Design review of the part built by this model. Coordinates are the model's own, in mm. A direction names the side the tool comes from. Coordinates: 2 decimals unless noted, no trailing zeros. Write each loop counter-clockwise with the first axis right and the second up, starting at its lowest first coordinate (ties: lowest second). Pieces come first, ordered by that corner, then holes. Notation, with made-up numbers: (24.5, 31) - (68.5, 31) arc R26 ccw to (68.5, 55) - close; hole circle Ø6 at (20, -32.75). An arc over 180 degrees is marked (long way). One line per item, written item: value.
from build123d import *

# Parameters (mm, degrees)
BOSS_EXTRUDE1_DEPTH                           = 3.175
SKETCH2_R                                     = 7.9375
CUT_EXTRUDE1_DEPTH                            = 3.175
CSK_FOR_4_FLAT_HEAD_SOCKET_CAP_SCREW1_A_COUNT = 2
CSK_FOR_4_FLAT_HEAD_SOCKET_CAP_SCREW1_A_PITCH = 44.901280605
CSK_FOR_4_FLAT_HEAD_SOCKET_CAP_SCRE_2_COUNT   = 2
CSK_FOR_4_FLAT_HEAD_SOCKET_CAP_SCRE_2_PITCH   = 44.901280605
CSK_FOR_4_FLAT_HEAD_SOCKET_CAP_SCRE_3_COUNT   = 2
CSK_FOR_4_FLAT_HEAD_SOCKET_CAP_SCRE_3_PITCH   = 81.964210025
CSK_FOR_4_FLAT_HEAD_SOCKET_CAP_SCRE_4_COUNT   = 2
CSK_FOR_4_FLAT_HEAD_SOCKET_CAP_SCRE_4_PITCH   = 81.964210025
SKETCH6_R                                     = 11.1125
SKETCH6_R_2                                   = 7.9375
BOSS_EXTRUDE2_DEPTH                           = 6.096
SKETCH7_R                                     = 8.73125
SKETCH7_R_2                                   = 6.35
BOSS_EXTRUDE3_DEPTH                           = 3.556
CUT_EXTRUDE2_START                            = -2.032
SKETCH8_R                                     = 6.35
CUT_EXTRUDE2_DEPTH                            = 2.032
FILLET1_R                                     = 3.175


with BuildPart() as part:
    # Sketch1 → Boss-Extrude1 (new body)
    with BuildSketch(Plane.XY):
        with BuildLine():
            Line((-34.925, 5.715), (-34.925, -41.275))
            Line((-34.925, -41.275), (34.925, -41.275))
            Line((34.925, -41.275), (34.925, 5.715))
            ThreePointArc((34.925, 5.715), (0, 40.64), (-34.925, 5.715))
        make_face()
    extrude(amount=BOSS_EXTRUDE1_DEPTH)

    # Sketch2 → Cut-Extrude1 (cut)
    with BuildSketch(Plane.XY.offset(3.175)):
        with Locations((0, 5.715)):
            Circle(SKETCH2_R)
    extrude(amount=-CUT_EXTRUDE1_DEPTH, mode=Mode.SUBTRACT)

    # Sketch5 → CSK for #4 Flat Head Socket Cap Screw1 (revolve, cut)
    with BuildSketch(Plane(origin=(0, 37.465, 3.175), x_dir=(0, -1, 0), z_dir=(1, 0, 0))):
        Polygon((0, 0), (0, 3.175), (1.63195, 3.175), (1.63195, 1.848124365), (3.2385, 0), align=None)
    csk_for_4_flat_head_socket_cap_screw1 = revolve(axis=Axis((0, 37.465, 9.525), (0, 0, -1)), mode=Mode.SUBTRACT)

    # CSK for #4 Flat Head Socket Cap Screw1 a: CSK for #4 Flat Head Socket Cap Screw1 ×2
    with Locations(*[Vector(-0.7071067811865475, -0.7071067811865476, 0) * (i * CSK_FOR_4_FLAT_HEAD_SOCKET_CAP_SCREW1_A_PITCH) for i in range(1, CSK_FOR_4_FLAT_HEAD_SOCKET_CAP_SCREW1_A_COUNT)]):
        add(csk_for_4_flat_head_socket_cap_screw1, mode=Mode.SUBTRACT)

    # CSK for _4 Flat Head Socket Cap Scre 2: CSK for #4 Flat Head Socket Cap Screw1 ×2
    with Locations(*[Vector(0.7071067811865475, -0.7071067811865477, 0) * (i * CSK_FOR_4_FLAT_HEAD_SOCKET_CAP_SCRE_2_PITCH) for i in range(1, CSK_FOR_4_FLAT_HEAD_SOCKET_CAP_SCRE_2_COUNT)]):
        add(csk_for_4_flat_head_socket_cap_screw1, mode=Mode.SUBTRACT)

    # CSK for _4 Flat Head Socket Cap Scre 3: CSK for #4 Flat Head Socket Cap Screw1 ×2
    with Locations(*[Vector(0.3873641921317683, -0.9219267772736089, 0) * (i * CSK_FOR_4_FLAT_HEAD_SOCKET_CAP_SCRE_3_PITCH) for i in range(1, CSK_FOR_4_FLAT_HEAD_SOCKET_CAP_SCRE_3_COUNT)]):
        add(csk_for_4_flat_head_socket_cap_screw1, mode=Mode.SUBTRACT)

    # CSK for _4 Flat Head Socket Cap Scre 4: CSK for #4 Flat Head Socket Cap Screw1 ×2
    with Locations(*[Vector(-0.3873641921317683, -0.9219267772736089, 0) * (i * CSK_FOR_4_FLAT_HEAD_SOCKET_CAP_SCRE_4_PITCH) for i in range(1, CSK_FOR_4_FLAT_HEAD_SOCKET_CAP_SCRE_4_COUNT)]):
        add(csk_for_4_flat_head_socket_cap_screw1, mode=Mode.SUBTRACT)

    # Sketch6 → Boss-Extrude2 (add)
    with BuildSketch(Plane(origin=(0, 0, 0), x_dir=(-1, 0, 0), z_dir=(0, 0, -1))):
        with Locations(Location((0, 5.715, 0), (0, 0, 180))):
            Circle(SKETCH6_R)
        with Locations(Location((0, 5.715, 0), (0, 0, 180))):
            Circle(SKETCH6_R_2, mode=Mode.SUBTRACT)
    extrude(amount=BOSS_EXTRUDE2_DEPTH)

    # Sketch7 → Boss-Extrude3 (add)
    with BuildSketch(Plane(origin=(0, 0, 0), x_dir=(-1, 0, 0), z_dir=(0, 0, -1))):
        with Locations(Location((15.875, -25.393519733, 0), (0, 0, 180))):
            Circle(SKETCH7_R)
        with Locations((15.875, -25.393519733)):
            Circle(SKETCH7_R_2, mode=Mode.SUBTRACT)
    extrude(amount=BOSS_EXTRUDE3_DEPTH)

    # Sketch8 → Cut-Extrude2 (cut)
    with BuildSketch(Plane(origin=(0, 0, 0), x_dir=(-1, 0, 0), z_dir=(0, 0, -1)).offset(CUT_EXTRUDE2_START)):
        with Locations((15.875, -25.393519733)):
            Circle(SKETCH8_R)
    extrude(amount=CUT_EXTRUDE2_DEPTH, mode=Mode.SUBTRACT)

    # Fillet1
    fillet1_edges = [part.edges().sort_by_distance(p)[0] for p in [
        (-11.1125, 5.715, 0),
        (-24.60625, -25.393519733, 0),
    ]]
    fillet(fillet1_edges, radius=FILLET1_R)


solid = part.part
1. Wall thickness on line 1 along X through (y, z) = (-38.1, 0.7) (3 decimals); line 2 along Y through (x, z) = (0, 0.5) (1 decimal); line 3 along Y through (x, z) = (1, 1.75) (3 decimals): over which ranges is each line inside the solid? List them lowest first.
Answer block:
line 1: x = -34.925 to -33.382, -30.118 to 30.118, 33.382 to 34.925
line 2: y = -41.3 to -2.2, 13.7 to 35.8, 39.1 to 40.6
line 3: y = -41.275 to -2.159, 13.589 to 35.733, 39.197 to 40.626
2. Consider section B-B, the plane y = -12. Write out the cut boundary in (x, z) (3 decimals).
Answer block:
outline: (-34.925, 0) - (34.925, 0) - (34.925, 3.175) - (-34.925, 3.175) - close
3. Consider section C-C, the plane y = 24. Write out the cut boundary in (x, z) (3 decimals).
Answer block:
outline: (-29.756, 0) - (29.756, 0) - (29.756, 3.175) - (-29.756, 3.175) - close
4. Mouldability with a two-part tool opening along Y and no side actions: class faces 4 (the face through (-33.468, 5.941, 1.442)), 5 (the face through (0, -41.275, 2)), 6 (the face through (0, -9, 3.175)) as released by +Y, released by -Y, zero draft, split by the parting line, or undercut.
Answer block:
face 4: undercut
face 5: released by -Y
face 6: zero draft
5. Insertion check: pin 1 Ø6.5 at (x, y) = (-13.5, -27) entering from -Z; pin 2 Ø1.5 at (x, y) = (26, -2.5) entering from -Z; pin 3 Ø3 at (x, y) = (-31.75, -38.1) entering from -Z; pin 4 Ø5 at (x, z) = (-6.5, -4) entering from -Y. Each pin has a flat end and moves straight along its axis. Give the tip position at first contact, or say it passes through.
Answer block:
pin 1: stops at z = 2.03
pin 2: stops at z = 0
pin 3: passes through
pin 4: stops at y = -30.72
6. Consider section A-A, the plane z = -2. Give the number of separate pieces and of enclosed holes in the cut face, then the cut area to 3 significant figures.
Answer block:
separate pieces: 2
enclosed holes: 2
area: 331 mm^2
7. For faces 1 (the face through (-8, -2, -5)), 2 (the face through (34.925, -18, 2)), 3 (the face through (-20, -20, -3.556)), list the 3-axis set-ups (+Z, -Z, +X, -X, +Y, -Y) from which the entire face can be reached by the end or side of a thin tool; tool diameter is ignored.
Answer block:
face 1: -Z
face 2: +Z, -Z, +X, +Y, -Y
face 3: -Z, +X, -X, -Y
